Can you work these out from the model? Positions are in its coordinate system, mm. A direction names the side the tool comes from. Coordinates: 2 decimals unless noted, no trailing zeros. Order: outer loops, then holes, each group sorted by start corner. A loop starts at its lowest first (then second) coordinate and runs counter-clockwise, first axis right, second up. Notation, with made-up numbers: (-20.5, 81) - (8.5, 81) arc R28 cw to (8.5, 118) - close; hole circle Ø4 at (81, -26). An arc over 180 degrees is marked (long way). Use a Markdown table: item, result. Add a question column.
(1) If I drill on L1, parallel to Y at x = 0, z = 19; L2, parallel to X at y = 0, z = 20, over which ranges is the centre line in solid material (lowest first)? Write a range as [from, to].
(2) On a 3-axis mill with a long thin cutter (end or side, diameter ignored), from which of +Z, -Z, +X, -X, +Y, -Y can I reach the whole of each face in a straight line? I mean faces 5 (the flat face through (16, -3.899, 23)), 6 (the flat face through (-16, -3.899, 23)), 7 (the cylindrical face through (-2.75, -12.4, 18.86)), 8 (the flat face through (-15.6, 0, 36.3)), 9 (the flat face through (15.6, 0, 36.3)). Say none if no direction works.
(3) I want a section at C-C (y = -7.5). List the corners of the cut face in (x, z) for me.
(4) I want a section at A-A (x = 0). List the corners of the cut face in (y, z) for me, and give its area (3 significant figures).
(5) We'd pull the mould along Y, two halves only. Please class faces 1 (the flat face through (16, 3.721, 23)), 2 (the flat face through (17, 0, 26.475)), 3 (the flat face through (0, 0, 0)), 4 (the flat face through (-15.6, -1.016, 36.3)): pulls with the +Y half, pulls with the -Y half, needs draft (parallel to the pull), parting line crosses it, or undercut.
(6) For pin 1 Ø2 at (x, z) = (-3, 3.5) entering from +Y; pin 2 Ø4 at (x, z) = (-13, 5.5) entering from -Y; pin 3 Ø5 at (x, z) = (-4, 18.5) entering from +Y, each with a flat end and sliding along its axis, tell me the tip position at first contact or that it passes through.
(7) I want a section at B-B (z = 9). List the corners of the cut face in (x, y) for me, and give its area (3 significant figures).
(8) I want a section at D-D (y = 3). List the corners of the cut face in (x, z) for me, and give its area (3 significant figures).
```python
from build123d import *

# Parameters (mm, degrees)
F0_W     = 15.24
F0_H     = 50.8
F2_W     = 7.62
F2_H     = 7.62
F3_DEPTH = 17.78
F5_W     = 0.762
F5_H     = 17.78
F6_DEPTH = 1.016
F8_R     = 12.7
F9_DEPTH = 51.562


# Not quite as in the source:
# - a feature names something its author has since deleted; it is built from what else it names


with BuildPart() as f1:
    # F0 (on Front) → F1 (revolve)
    with BuildSketch(Plane.XZ):
        with Locations((-7.62, 12.8494124473)):
            Rectangle(F0_W, F0_H)
    revolve(axis=Axis((0, 0, 12.8494124473), (0, 0, -1)))

    # F2 (on Right) → F3 (join)
    with BuildSketch(Plane.YZ):
        with Locations((-0.0885345507, 22.6649723111)):
            Rectangle(F2_W, F2_H)
    extrude(amount=F3_DEPTH)

    # F4: F1 across plane


with BuildPart() as f1_1:
    add(f1.part)
    add(f1.part.mirror(Plane.YZ))

    # F5 (on Front) → F6 (join)
    with BuildSketch(Plane.XZ):
        Polygon((15.2397256883, 44.2549723111), (16.0017256883, 44.2549723111), (16.6367256883, 44.2549723111), (16.6367256883, 45.9895022213), (16.2511286259, 45.9895022213), (16.2511286259, 44.5822738111), (14.9926585078, 44.5822738111), (14.9926585078, 45.9895022213), (14.6047256883, 45.9895022213), (14.6047256883, 44.2549723111), align=None)
        with Locations((15.6207256883, 35.3649723111)):
            Rectangle(F5_W, F5_H)
    extrude(amount=F6_DEPTH)

    # F7: F1 across plane


with BuildPart() as f1_2:
    add(f1_1.part)
    add(f1_1.part.mirror(Plane.YZ))

    # F8 (on Top) → F9 (cut)
    with BuildSketch(Plane.XY):
        Circle(F8_R)
    extrude(amount=F9_DEPTH, mode=Mode.SUBTRACT)


solid = f1_2.part
```
Answers follow:
| question | item | result |
|---|---|---|
| 1 | L1 | y = [-15.24, -12.7], [12.7, 15.24] |
| 1 | L2 | x = [-17.78, -12.7], [12.7, 17.78] |
| 2 | face 5 | +Z, -Z, +X, -Y |
| 2 | face 6 | +Z, -Z, -X, -Y |
| 2 | face 7 | +Z |
| 2 | face 8 | +Z, -X, +Y |
| 2 | face 9 | +Z, +X, +Y |
| 3 | outline | (-13.27, -12.55) - (13.27, -12.55) - (13.27, 38.25) - (10.25, 38.25) - (10.25, 0) - (-10.25, 0) - (-10.25, 38.25) - (-13.27, 38.25) - close |
| 4 | outline | (-15.24, -12.55) - (15.24, -12.55) - (15.24, 38.25) - (12.7, 38.25) - (12.7, 0) - (-12.7, 0) - (-12.7, 38.25) - (-15.24, 38.25) - close |
| 4 | area | 577 mm² |
| 5 | face 1 | pulls with the +Y half |
| 5 | face 2 | needs draft |
| 5 | face 3 | undercut |
| 5 | face 4 | pulls with the -Y half |
| 6 | pin 1 | stops at y = 15.11 |
| 6 | pin 2 | stops at y = -10.55 |
| 6 | pin 3 | stops at y = 15.17 |
| 7 | outline | circle Ø30.48 at (0, 0); hole circle Ø25.4 at (0, 0) |
| 7 | area | 223 mm² |
| 8 | outline | (-17.78, 18.85) - (-14.94, 18.85) - (-14.94, -12.55) - (14.94, -12.55) - (14.94, 18.85) - (17.78, 18.85) - (17.78, 26.47) - (14.94, 26.47) - (14.94, 38.25) - (12.34, 38.25) - (12.34, 0) - (-12.34, 0) - (-12.34, 38.25) - (-14.94, 38.25) - (-14.94, 26.47) - (-17.78, 26.47) - close |
| 8 | area | 617 mm² |
